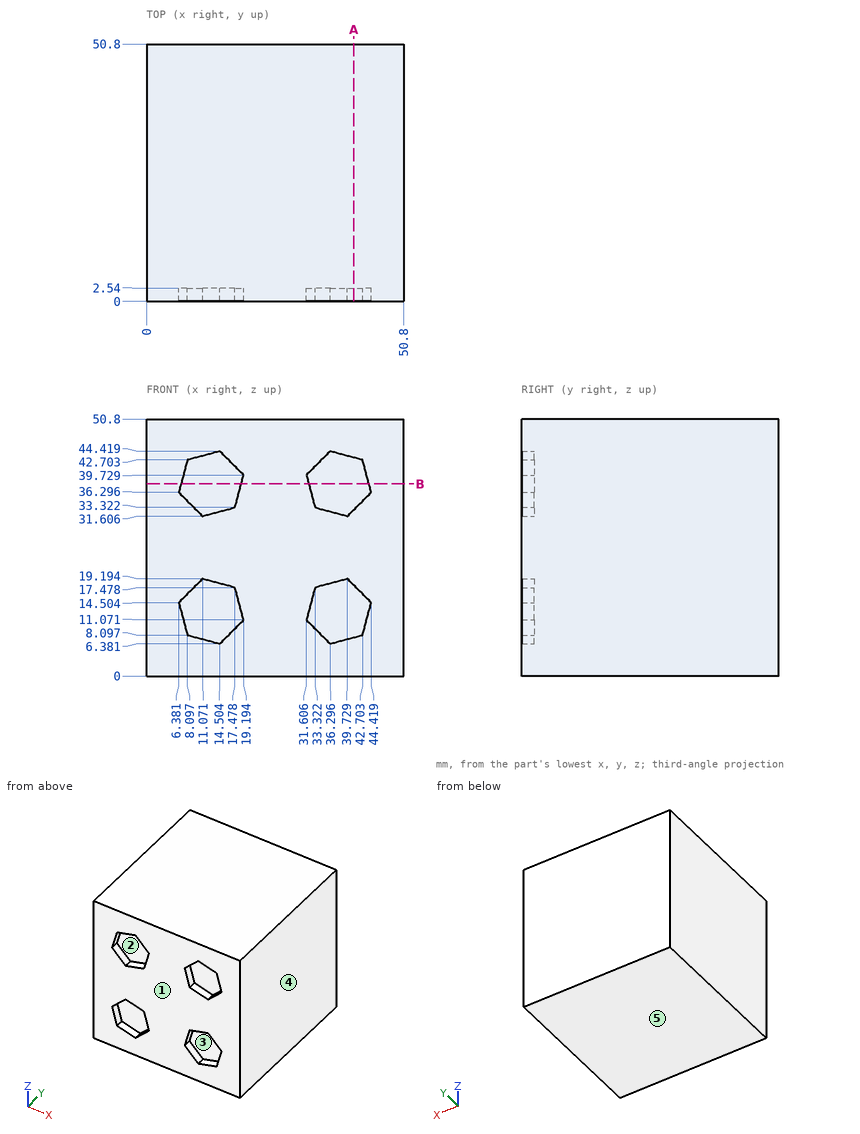
Job drawing, mm, ordinate dimensions from the low corner. One solid piece. A direction names the side the tool comes from. Coordinates: 2 decimals unless noted, no trailing zeros. Write each loop counter-clockwise with the first axis right and the second up, starting at its lowest first coordinate (ties: lowest second). Pieces come first, ordered by that corner, then holes.
Item 1: Probe line 1 (Y direction, x = 12, z = 33). List the from-to ranges inside material, lowest first.
Item 2: Mould opens along Z. For the marked faces 3, 4 and 5 say: released by +Z, released by -Z, zero draft, split by the parting line, or undercut.
Item 3: Slice it at A-A (x = 41). Write the cut outline in (y, z).
Item 4: Which spindle directions (+Z, -Z, +X, -X, +Y, -Y) get a long thin tool onto all of the face, cutting with end or side? Do the marked faces 1 and 2. Say none if no direction does.
Item 5: Slice it at B-B (z = 38). Write the cut outline in (x, y), and give its area (3 significant figures).
Results found:
1. line 1: y = 2.54 to 50.8
2. face 3: undercut
2. face 4: zero draft
2. face 5: released by -Z
3. outline: (0, 0) - (50.8, 0) - (50.8, 50.8) - (0, 50.8) - (0, 43.16) - (2.54, 43.16) - (2.54, 32.88) - (0, 32.88) - (0, 17.92) - (2.54, 17.92) - (2.54, 7.64) - (0, 7.64) - close
4. face 1: +Z, -Z, +X, -X, -Y
4. face 2: -Y
5. outline: (0, 0) - (6.84, 0) - (6.84, 2.54) - (18.73, 2.54) - (18.73, 0) - (32.07, 0) - (32.07, 2.54) - (43.96, 2.54) - (43.96, 0) - (50.8, 0) - (50.8, 50.8) - (0, 50.8) - close
5. area: 2,520 mm2
